Here's the drawing with two shaded views (mm, measured from the low corner). I have some questions. Round coordinates to 2 decimals unless told otherwise and drop trailing zeros. Loops run counter-clockwise (first coordinate to the right, second up) from the corner with the lowest first, then second, coordinate; pieces in that order, holes last.
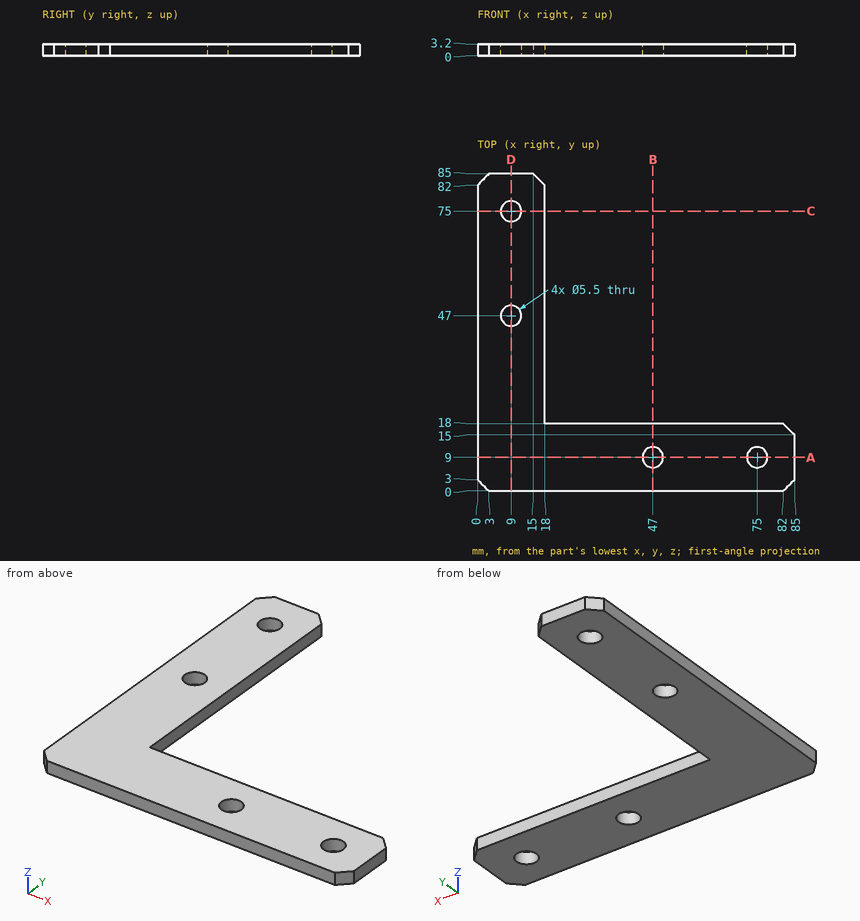
Item 1: If I drill on line 1 along Y through (x, z) = (9, 1.9); line 2 along Y through (x, z) = (47, 2.1); line 3 along Y through (x, z) = (34, 1.25), over which ranges is the centre line in solid material (lowest first)?
Results list:
line 1: y = 0 to 44.25, 49.75 to 72.25, 77.75 to 85
line 2: y = 0 to 6.25, 11.75 to 18
line 3: y = 0 to 18
Item 2: Will this pin go through, and if not, where does the flat tip stop? pin 1 (12 mm diameter, centred on x = 72, y = 26.5, fed in from -Z).
Results list:
pin 1: passes through
Item 3: If we section it at A-A, the plane y = 9: Please give me the cut outline in (x, z), then the cut area to 3 significant figures.
Results list:
outline: (0, 0) - (44.25, 0) - (44.25, 3.2) - (0, 3.2) - close; (49.75, 0) - (72.25, 0) - (72.25, 3.2) - (49.75, 3.2) - close; (77.75, 0) - (85, 0) - (85, 3.2) - (77.75, 3.2) - close
area: 237 mm2
Item 4: If we section it at B-B, the plane x = 47: Please give me the cut outline in (y, z).
Results list:
outline: (0, 0) - (6.25, 0) - (6.25, 3.2) - (0, 3.2) - close; (11.75, 0) - (18, 0) - (18, 3.2) - (11.75, 3.2) - close
